Read the model definition and answer for the solid it produces. Units are mm, in the model's axes. Face numbers are marked on the shaded views. Round coordinates to 2 decimals unless told otherwise and drop trailing zeros. Order: outer loops, then holes, each group sorted by start corner. A loop starts at its lowest first (then second) coordinate and runs counter-clockwise, first axis right, second up. Notation, with made-up numbers: (3, 78) -> (43, 78) arc R8 ccw to (43, 90) -> close; hole circle Ø11 at (28.5, 27). An arc over 180 degrees is marked (long way). Answer as a JSON object with one key per item and string values. Group by question number.
Item 1: Section B-B, the plane y = 3.35 is taken. Count the separate pieces of the cut face and the enclosed holes in it, plus the area to 3 significant figures.
Item 2: Consider probe 1 along X at (y, z) = (2.8, 132); probe 2 along X at (y, z) = (3.5, 0); probe 3 along Z at (x, y) = (3.5, 4.55). Determine where each line is inside the solid, lowest interval first. Write a range as from..to.
Item 3: Section A-A, the plane x = -8 is taken. Write down the section's boundary in (y, z).
Item 4: The mould has two halves that part along Y. Classify the marked faces 1 and 2: pulls with the +Y half, pulls with the -Y half, needs draft (parallel to the pull), parting line crosses it, or undercut.
Item 5: Given P1, Ø2.5, axis at x = -40, z = -100, coming from the -Y side, flat-ended and moving along its own axis, determine where the tip first touches the part or whether it passes through.
from build123d import *

# Parameters (mm, degrees)
SKETCH_1_R      = 1.7
SKETCH_1_R_2    = 2
SKETCH_1_R_3    = 2.5
EXTRUDE_2_DEPTH = 5


with BuildPart() as part:
    # 草图1 → 凸台-拉伸2 (new body)
    with BuildSketch(Plane(origin=(0, 0, 0), x_dir=(1, 0, 0), z_dir=(0, 1, 0))):
        with BuildLine():
            ThreePointArc((-65, 160), (-68.535533906, 158.535533906), (-70, 155))
            Line((-70, 155), (-70, 120))
            Line((-70, 120), (-70, 0))
            Line((-70, 0), (-70, -155))
            ThreePointArc((-70, -155), (-68.535533906, -158.535533906), (-65, -160))
            Line((-65, -160), (65, -160))
            ThreePointArc((65, -160), (68.535533906, -158.535533906), (70, -155))
            Line((70, -155), (70, 20))
            Line((70, 20), (70, 155))
            ThreePointArc((70, 155), (68.535533906, 158.535533906), (65, 160))
            Line((65, 160), (-65, 160))
        make_face()
        with Locations(Location((-62, -148, 0), (0, 0, 270))):
            Circle(SKETCH_1_R, mode=Mode.SUBTRACT)
        with Locations(Location((-48, -148, 0), (0, 0, 270))):
            Circle(SKETCH_1_R, mode=Mode.SUBTRACT)
        with Locations(Location((-62, -132, 0), (0, 0, 270))):
            Circle(SKETCH_1_R, mode=Mode.SUBTRACT)
        with Locations(Location((-60, -120, 0), (0, 0, 270))):
            Circle(SKETCH_1_R_2, mode=Mode.SUBTRACT)
        with Locations(Location((-48, -132, 0), (0, 0, 270))):
            Circle(SKETCH_1_R, mode=Mode.SUBTRACT)
        with Locations(Location((-35, -150, 0), (0, 0, 270))):
            Circle(SKETCH_1_R_3, mode=Mode.SUBTRACT)
        with Locations(Location((-60, -100, 0), (0, 0, 270))):
            Circle(SKETCH_1_R_2, mode=Mode.SUBTRACT)
        with Locations(Location((-60, -80, 0), (0, 0, 270))):
            Circle(SKETCH_1_R_2, mode=Mode.SUBTRACT)
        with Locations(Location((-40, -100, 0), (0, 0, 270))):
            Circle(SKETCH_1_R_2, mode=Mode.SUBTRACT)
        with Locations(Location((-40, -80, 0), (0, 0, 270))):
            Circle(SKETCH_1_R_2, mode=Mode.SUBTRACT)
        with BuildLine():
            Line((-20, -125), (20, -125))
            ThreePointArc((20, -125), (23.535533906, -126.464466094), (25, -130))
            Line((25, -130), (25, -150))
            ThreePointArc((25, -150), (23.535533906, -153.535533906), (20, -155))
            Line((20, -155), (-20, -155))
            ThreePointArc((-20, -155), (-23.535533906, -153.535533906), (-25, -150))
            Line((-25, -150), (-25, -130))
            ThreePointArc((-25, -130), (-23.535533906, -126.464466094), (-20, -125))
        make_face(mode=Mode.SUBTRACT)
        with Locations(Location((-20, -100, 0), (0, 0, 270))):
            Circle(SKETCH_1_R_2, mode=Mode.SUBTRACT)
        with Locations(Location((-20, -80, 0), (0, 0, 270))):
            Circle(SKETCH_1_R_2, mode=Mode.SUBTRACT)
        with Locations(Location((0, -100, 0), (0, 0, 270))):
            Circle(SKETCH_1_R_2, mode=Mode.SUBTRACT)
        with Locations(Location((0, -80, 0), (0, 0, 270))):
            Circle(SKETCH_1_R_2, mode=Mode.SUBTRACT)
        with Locations(Location((-60, -60, 0), (0, 0, 270))):
            Circle(SKETCH_1_R_2, mode=Mode.SUBTRACT)
        with Locations(Location((-60, -40, 0), (0, 0, 270))):
            Circle(SKETCH_1_R_2, mode=Mode.SUBTRACT)
        with Locations(Location((-40, -60, 0), (0, 0, 270))):
            Circle(SKETCH_1_R_2, mode=Mode.SUBTRACT)
        with Locations(Location((-40, -40, 0), (0, 0, 270))):
            Circle(SKETCH_1_R_2, mode=Mode.SUBTRACT)
        with Locations(Location((-60, -20, 0), (0, 0, 270))):
            Circle(SKETCH_1_R_2, mode=Mode.SUBTRACT)
        with Locations(Location((-40, -20, 0), (0, 0, 270))):
            Circle(SKETCH_1_R_2, mode=Mode.SUBTRACT)
        with Locations(Location((-20, -60, 0), (0, 0, 270))):
            Circle(SKETCH_1_R_2, mode=Mode.SUBTRACT)
        with Locations(Location((-20, -40, 0), (0, 0, 270))):
            Circle(SKETCH_1_R_2, mode=Mode.SUBTRACT)
        with Locations(Location((0, -60, 0), (0, 0, 270))):
            Circle(SKETCH_1_R_2, mode=Mode.SUBTRACT)
        with Locations(Location((0, -40, 0), (0, 0, 270))):
            Circle(SKETCH_1_R_2, mode=Mode.SUBTRACT)
        with Locations(Location((-20, -20, 0), (0, 0, 270))):
            Circle(SKETCH_1_R_2, mode=Mode.SUBTRACT)
        with Locations(Location((0, -20, 0), (0, 0, 270))):
            Circle(SKETCH_1_R_2, mode=Mode.SUBTRACT)
        with Locations(Location((20, -100, 0), (0, 0, 270))):
            Circle(SKETCH_1_R_2, mode=Mode.SUBTRACT)
        with Locations(Location((20, -80, 0), (0, 0, 270))):
            Circle(SKETCH_1_R_2, mode=Mode.SUBTRACT)
        with Locations(Location((35, -150, 0), (0, 0, 270))):
            Circle(SKETCH_1_R_3, mode=Mode.SUBTRACT)
        with Locations(Location((48, -148, 0), (0, 0, 270))):
            Circle(SKETCH_1_R, mode=Mode.SUBTRACT)
        with Locations(Location((62, -148, 0), (0, 0, 270))):
            Circle(SKETCH_1_R, mode=Mode.SUBTRACT)
        with Locations(Location((48, -132, 0), (0, 0, 270))):
            Circle(SKETCH_1_R, mode=Mode.SUBTRACT)
        with Locations(Location((62, -132, 0), (0, 0, 270))):
            Circle(SKETCH_1_R, mode=Mode.SUBTRACT)
        with Locations(Location((60, -120, 0), (0, 0, 270))):
            Circle(SKETCH_1_R_2, mode=Mode.SUBTRACT)
        with Locations(Location((40, -100, 0), (0, 0, 270))):
            Circle(SKETCH_1_R_2, mode=Mode.SUBTRACT)
        with Locations(Location((40, -80, 0), (0, 0, 270))):
            Circle(SKETCH_1_R_2, mode=Mode.SUBTRACT)
        with Locations(Location((60, -100, 0), (0, 0, 270))):
            Circle(SKETCH_1_R_2, mode=Mode.SUBTRACT)
        with Locations(Location((60, -80, 0), (0, 0, 270))):
            Circle(SKETCH_1_R_2, mode=Mode.SUBTRACT)
        with Locations(Location((20, -60, 0), (0, 0, 270))):
            Circle(SKETCH_1_R_2, mode=Mode.SUBTRACT)
        with Locations(Location((20, -40, 0), (0, 0, 270))):
            Circle(SKETCH_1_R_2, mode=Mode.SUBTRACT)
        with Locations(Location((20, -20, 0), (0, 0, 270))):
            Circle(SKETCH_1_R_2, mode=Mode.SUBTRACT)
        with Locations(Location((40, -60, 0), (0, 0, 270))):
            Circle(SKETCH_1_R_2, mode=Mode.SUBTRACT)
        with Locations(Location((40, -40, 0), (0, 0, 270))):
            Circle(SKETCH_1_R_2, mode=Mode.SUBTRACT)
        with Locations(Location((60, -60, 0), (0, 0, 270))):
            Circle(SKETCH_1_R_2, mode=Mode.SUBTRACT)
        with Locations(Location((60, -40, 0), (0, 0, 270))):
            Circle(SKETCH_1_R_2, mode=Mode.SUBTRACT)
        with Locations(Location((40, -20, 0), (0, 0, 270))):
            Circle(SKETCH_1_R_2, mode=Mode.SUBTRACT)
        with Locations(Location((60, -20, 0), (0, 0, 270))):
            Circle(SKETCH_1_R_2, mode=Mode.SUBTRACT)
        with Locations(Location((-60, 0, 0), (0, 0, 270))):
            Circle(SKETCH_1_R_2, mode=Mode.SUBTRACT)
        with Locations(Location((-60, 20, 0), (0, 0, 270))):
            Circle(SKETCH_1_R_2, mode=Mode.SUBTRACT)
        with Locations(Location((-40, 20, 0), (0, 0, 270))):
            Circle(SKETCH_1_R_2, mode=Mode.SUBTRACT)
        with Locations(Location((-60, 40, 0), (0, 0, 270))):
            Circle(SKETCH_1_R_2, mode=Mode.SUBTRACT)
        with Locations(Location((-60, 60, 0), (0, 0, 270))):
            Circle(SKETCH_1_R_2, mode=Mode.SUBTRACT)
        with Locations(Location((-40, 40, 0), (0, 0, 270))):
            Circle(SKETCH_1_R_2, mode=Mode.SUBTRACT)
        with Locations(Location((-40, 60, 0), (0, 0, 270))):
            Circle(SKETCH_1_R_2, mode=Mode.SUBTRACT)
        with Locations(Location((-20, 20, 0), (0, 0, 270))):
            Circle(SKETCH_1_R_2, mode=Mode.SUBTRACT)
        with Locations(Location((0, 20, 0), (0, 0, 270))):
            Circle(SKETCH_1_R_2, mode=Mode.SUBTRACT)
        with Locations(Location((-20, 40, 0), (0, 0, 270))):
            Circle(SKETCH_1_R_2, mode=Mode.SUBTRACT)
        with Locations(Location((-20, 60, 0), (0, 0, 270))):
            Circle(SKETCH_1_R_2, mode=Mode.SUBTRACT)
        with Locations(Location((0, 40, 0), (0, 0, 270))):
            Circle(SKETCH_1_R_2, mode=Mode.SUBTRACT)
        with Locations(Location((0, 60, 0), (0, 0, 270))):
            Circle(SKETCH_1_R_2, mode=Mode.SUBTRACT)
        with Locations(Location((-60, 80, 0), (0, 0, 270))):
            Circle(SKETCH_1_R_2, mode=Mode.SUBTRACT)
        with Locations(Location((-60, 100, 0), (0, 0, 270))):
            Circle(SKETCH_1_R_2, mode=Mode.SUBTRACT)
        with Locations(Location((-40, 80, 0), (0, 0, 270))):
            Circle(SKETCH_1_R_2, mode=Mode.SUBTRACT)
        with Locations(Location((-40, 100, 0), (0, 0, 270))):
            Circle(SKETCH_1_R_2, mode=Mode.SUBTRACT)
        with BuildLine():
            ThreePointArc((-58, 120), (-60, 118), (-62, 120))
            ThreePointArc((-62, 120), (-60, 122), (-58, 120))
        make_face(mode=Mode.SUBTRACT)
        with Locations(Location((-62, 132, 0), (0, 0, 270))):
            Circle(SKETCH_1_R, mode=Mode.SUBTRACT)
        with Locations(Location((-48, 132, 0), (0, 0, 270))):
            Circle(SKETCH_1_R, mode=Mode.SUBTRACT)
        with Locations(Location((-62, 148, 0), (0, 0, 270))):
            Circle(SKETCH_1_R, mode=Mode.SUBTRACT)
        with Locations(Location((-48, 148, 0), (0, 0, 270))):
            Circle(SKETCH_1_R, mode=Mode.SUBTRACT)
        with Locations(Location((-35, 150, 0), (0, 0, 270))):
            Circle(SKETCH_1_R_3, mode=Mode.SUBTRACT)
        with Locations(Location((-20, 80, 0), (0, 0, 270))):
            Circle(SKETCH_1_R_2, mode=Mode.SUBTRACT)
        with Locations(Location((-20, 100, 0), (0, 0, 270))):
            Circle(SKETCH_1_R_2, mode=Mode.SUBTRACT)
        with Locations(Location((0, 80, 0), (0, 0, 270))):
            Circle(SKETCH_1_R_2, mode=Mode.SUBTRACT)
        with Locations(Location((0, 100, 0), (0, 0, 270))):
            Circle(SKETCH_1_R_2, mode=Mode.SUBTRACT)
        with BuildLine():
            ThreePointArc((-20, 125), (-23.535533906, 126.464466094), (-25, 130))
            Line((-25, 130), (-25, 150))
            ThreePointArc((-25, 150), (-23.535533906, 153.535533906), (-20, 155))
            Line((-20, 155), (20, 155))
            ThreePointArc((20, 155), (23.535533906, 153.535533906), (25, 150))
            Line((25, 150), (25, 130))
            ThreePointArc((25, 130), (23.535533906, 126.464466094), (20, 125))
            Line((20, 125), (-20, 125))
        make_face(mode=Mode.SUBTRACT)
        with Locations(Location((20, 20, 0), (0, 0, 270))):
            Circle(SKETCH_1_R_2, mode=Mode.SUBTRACT)
        with Locations(Location((20, 40, 0), (0, 0, 270))):
            Circle(SKETCH_1_R_2, mode=Mode.SUBTRACT)
        with Locations(Location((20, 60, 0), (0, 0, 270))):
            Circle(SKETCH_1_R_2, mode=Mode.SUBTRACT)
        with Locations(Location((40, 20, 0), (0, 0, 270))):
            Circle(SKETCH_1_R_2, mode=Mode.SUBTRACT)
        with Locations(Location((60, 0, 0), (0, 0, 270))):
            Circle(SKETCH_1_R_2, mode=Mode.SUBTRACT)
        with Locations(Location((60, 20, 0), (0, 0, 270))):
            Circle(SKETCH_1_R_2, mode=Mode.SUBTRACT)
        with Locations(Location((40, 40, 0), (0, 0, 270))):
            Circle(SKETCH_1_R_2, mode=Mode.SUBTRACT)
        with Locations(Location((40, 60, 0), (0, 0, 270))):
            Circle(SKETCH_1_R_2, mode=Mode.SUBTRACT)
        with Locations(Location((60, 40, 0), (0, 0, 270))):
            Circle(SKETCH_1_R_2, mode=Mode.SUBTRACT)
        with Locations(Location((60, 60, 0), (0, 0, 270))):
            Circle(SKETCH_1_R_2, mode=Mode.SUBTRACT)
        with Locations(Location((20, 80, 0), (0, 0, 270))):
            Circle(SKETCH_1_R_2, mode=Mode.SUBTRACT)
        with Locations(Location((20, 100, 0), (0, 0, 270))):
            Circle(SKETCH_1_R_2, mode=Mode.SUBTRACT)
        with Locations(Location((40, 80, 0), (0, 0, 270))):
            Circle(SKETCH_1_R_2, mode=Mode.SUBTRACT)
        with Locations(Location((40, 100, 0), (0, 0, 270))):
            Circle(SKETCH_1_R_2, mode=Mode.SUBTRACT)
        with Locations(Location((60, 80, 0), (0, 0, 270))):
            Circle(SKETCH_1_R_2, mode=Mode.SUBTRACT)
        with Locations(Location((60, 100, 0), (0, 0, 270))):
            Circle(SKETCH_1_R_2, mode=Mode.SUBTRACT)
        with Locations(Location((35, 150, 0), (0, 0, 270))):
            Circle(SKETCH_1_R_3, mode=Mode.SUBTRACT)
        with Locations(Location((48, 132, 0), (0, 0, 270))):
            Circle(SKETCH_1_R, mode=Mode.SUBTRACT)
        with Locations(Location((60, 120, 0), (0, 0, 270))):
            Circle(SKETCH_1_R_2, mode=Mode.SUBTRACT)
        with Locations(Location((62, 132, 0), (0, 0, 270))):
            Circle(SKETCH_1_R, mode=Mode.SUBTRACT)
        with Locations(Location((48, 148, 0), (0, 0, 270))):
            Circle(SKETCH_1_R, mode=Mode.SUBTRACT)
        with Locations(Location((62, 148, 0), (0, 0, 270))):
            Circle(SKETCH_1_R, mode=Mode.SUBTRACT)
    extrude(amount=EXTRUDE_2_DEPTH)


solid = part.part
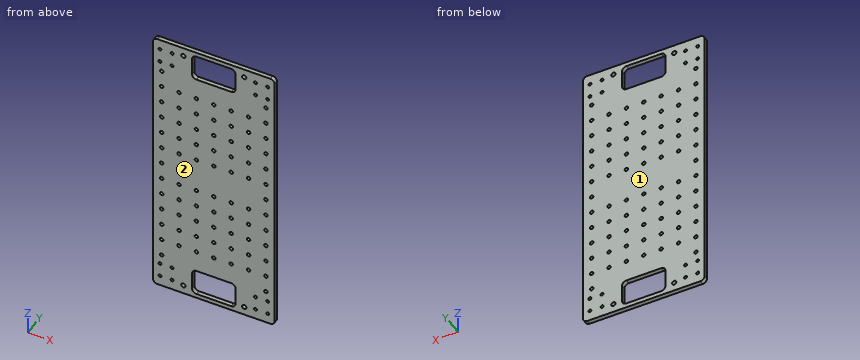
Values found:
{
 "1": {"separate pieces": "1", "enclosed holes": "98", "area": "40,600 mm2"},
 "2": {"probe 1": "-70..-63.7, -60.3..-49.7, -46.3..-25, 25..46.3, 49.7..60.3, 63.7..70", "probe 2": "-70..-62, -58..58, 62..70", "probe 3": "-160..-155, -125..125, 155..160"},
 "3": {"outline": "(0, -160) -> (5, -160) -> (5, -155) -> (0, -155) -> close; (0, -125) -> (5, -125) -> (5, 125) -> (0, 125) -> close; (0, 155) -> (5, 155) -> (5, 160) -> (0, 160) -> close"},
 "4": {"face 1": "pulls with the +Y half", "face 2": "pulls with the -Y half"},
 "5": {"P1": "through"}
}
